The listing builds one solid part. Answer for the finished solid, in the listing's coordinates (mm). Face numbers are marked on the shaded views. A direction names the side the tool comes from. Give positions to 0.01 mm unless a question says otherwise; leave off trailing zeros. Write each loop counter-clockwise with the first axis right and the second up, starting at its lowest first coordinate (ties: lowest second). Pieces come first, ordered by that corner, then holes.
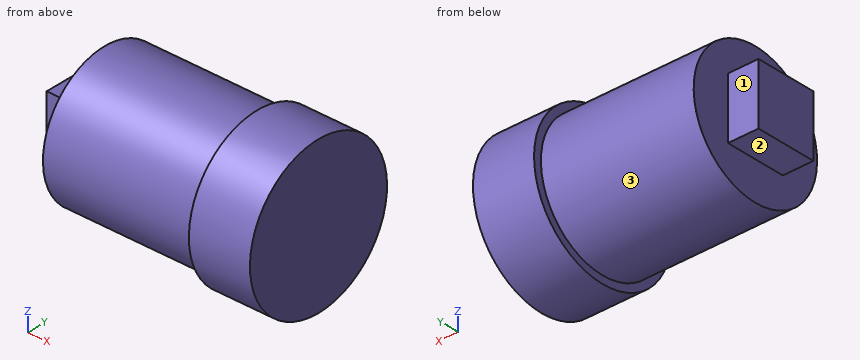
```python
from build123d import *

# Parameters (mm, degrees)
SKETCH_1_R      = 25
EXTRUDE_1_DEPTH = 20
SKETCH_2_W      = 20
SKETCH_2_H      = 20
EXTRUDE_2_DEPTH = 60
SKETCH_3_R      = 22.5
EXTRUDE_3_DEPTH = 50


with BuildPart() as part:
    # 草图1 → 凸台-拉伸1 (new body)
    with BuildSketch(Plane(origin=(0, 0, 0), x_dir=(0, 0, -1), z_dir=(1, 0, 0))):
        Circle(SKETCH_1_R)
    extrude(amount=EXTRUDE_1_DEPTH)

    # 草图2 → 凸台-拉伸2 (add)
    with BuildSketch(Plane.ZY):
        Rectangle(SKETCH_2_W, SKETCH_2_H)
    extrude(amount=EXTRUDE_2_DEPTH)

    # 草图3 → 凸台-拉伸3 (add)
    with BuildSketch(Plane.ZY):
        with Locations(Location((0, 0, 0), (0, 0, 180))):
            Circle(SKETCH_3_R)
    extrude(amount=EXTRUDE_3_DEPTH)


solid = part.part
```
Item 1: Each of these flat-tipped pins is pushed along its axis until it touches: P1, Ø3, axis at x = -50.5, y = 4.5, coming from the -Z side; P2, Ø5, axis at x = -54.5, y = 4, coming from the -Z side; P3, Ø10, axis at x = -48, z = -2, coming from the -Y side. Where does it stop, or does it pass through?
Conclusion:
P1: stops at z = -22.29
P2: stops at z = -10
P3: stops at y = -22.5
Item 2: Consider probe 1 along X at (y, z) = (-10.5, 2); probe 2 along X at (y, z) = (15, 18); probe 3 along Y at (x, z) = (-32.5, -6.5). Determine where each line is inside the solid, lowest interval first.
Conclusion:
probe 1: x = -50 to 20
probe 2: x = 0 to 20
probe 3: y = -21.54 to 21.54
Item 3: A cutting plane is placed at D-D, the plane z = -16.5. Give the vertices of the cut face in (x, y), plus the area to 3 significant figures.
Conclusion:
outline: (-50, -15.3) - (0, -15.3) - (0, -18.78) - (20, -18.78) - (20, 18.78) - (0, 18.78) - (0, 15.3) - (-50, 15.3) - close
area: 2,280 mm2
Item 4: Which of the six approach directions +Z, -Z, +X, -X, +Y, -Y give full straight-line access (tool end or side, diameter ignored) to the marked faces 1, 2 and 3?
Conclusion:
face 1: +Z, -Z, -X, +Y
face 2: -Z, -X, +Y, -Y
face 3: -X
Item 5: A cutting plane is placed at A-A, the plane z = 0. Give the vertices of the cut face in (x, y).
Conclusion:
outline: (-60, -10) - (-50, -10) - (-50, -22.5) - (0, -22.5) - (0, -25) - (20, -25) - (20, 25) - (0, 25) - (0, 22.5) - (-50, 22.5) - (-50, 10) - (-60, 10) - close
Item 6: A cutting plane is placed at C-C, the plane x = 9.5. Give the vertices of the cut face in (y, z).
Conclusion:
outline: circle Ø50 at (0, 0)
